Here's how the part is built. I have some questions about the finished solid (model axes, mm). Face numbers are marked on the shaded views. A direction names the side the tool comes from. Coordinates: 2 decimals unless noted, no trailing zeros. Write each loop counter-clockwise with the first axis right and the second up, starting at its lowest first coordinate (ties: lowest second). Pieces come first, ordered by that corner, then holes. Notation, with made-up numbers: (-26, -39) -> (31, -39) arc R18 cw to (31, -15) -> close; hole circle Ø3 at (10, -32.75). An arc over 180 degrees is marked (long way). Put each result on its own line as item: value. Start each with the question number.
Item 1: I need wall thicknesses on line 1 (X direction, y = 17.5, z = 2.5); line 2 (Y direction, x = 0, z = 0.2); line 3 (Y direction, x = 7.5, z = 6.25). Which ranges of each line are inside material? Lowest first, please. Write a range as [from, to].
Item 2: I want a section at A-A, the plane x = 3. List the corners of the cut face in (y, z) for me, then the cut area to 3 significant figures.
Item 3: For pin 1 (11.5 mm diameter, centred on x = 0, y = 17, fed in from +Z); pin 2 (1.3 mm diameter, centred on x = -13, z = 3, fed in from -Y), each with a flat end and sliding along its axis, tell me the tip position at first contact or that it passes through.
Item 4: If we mould it in two halves opening along Y, with no side actions, what happens to the marked faces 3, 4, 5 and 6? For each: released by +Y, released by -Y, zero draft, split by the parting line, or undercut.
Item 5: On a 3-axis mill with a long thin cutter (end or side, diameter ignored), from which of +Z, -Z, +X, -X, +Y, -Y can I reach the whole of each face in a straight line? I mean the marked faces 1 and 2. Say none if no direction works.
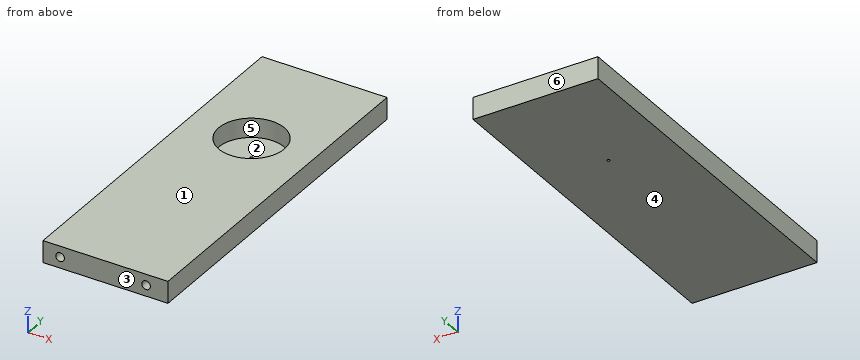
from build123d import *

# Parameters (mm, degrees)
SKETCH1_W                       = 36.27882
SKETCH1_H                       = 102.003225
EXTRUDE1_DEPTH                  = 6.35
SKETCH2_R                       = 9.525
EXTRUDE2_DEPTH                  = 5.588
SKETCH3_R                       = 0.396875
EXTRUDE3_DEPTH                  = 55.419007863
F_3_48_TAPPED_HOLE1_D           = 1.9939
F_3_48_TAPPED_HOLE1_DEPTH       = 9.144
F_3_48_TAPPED_HOLE1_CBORE_D     = 2.5146
F_3_48_TAPPED_HOLE1_CBORE_DEPTH = 7.62
F_3_48_TAPPED_HOLE1_TIP         = 0.599027994


with BuildPart() as part:
    # Sketch1 → Extrude1 (new body)
    with BuildSketch(Plane.XY):
        Rectangle(SKETCH1_W, SKETCH1_H)
    extrude(amount=EXTRUDE1_DEPTH)

    # Sketch2 → Extrude2 (cut)
    with BuildSketch(Plane.XY.offset(6.35)):
        with Locations((0, 17.0005375)):
            Circle(SKETCH2_R)
    extrude(amount=-EXTRUDE2_DEPTH, mode=Mode.SUBTRACT)

    # Sketch3 → Extrude3 (cut, through all)
    with BuildSketch(Plane.XY.offset(0.762)):
        with Locations((0, 17.0005375)):
            Circle(SKETCH3_R)
    extrude(amount=-EXTRUDE3_DEPTH, mode=Mode.SUBTRACT)

    # #3-48 Tapped Hole1
    with Locations(Plane(origin=(-14.071004552, -51.0016125, -59.648711207), x_dir=(0, 0, -1), z_dir=(0, -1, 0))):
        with Locations((-62.823711207, 25.860414552), (-62.823711207, 0.892214552)):
            CounterBoreHole(F_3_48_TAPPED_HOLE1_D / 2, F_3_48_TAPPED_HOLE1_CBORE_D / 2, F_3_48_TAPPED_HOLE1_CBORE_DEPTH, depth=F_3_48_TAPPED_HOLE1_DEPTH)
            with Locations((0, 0, -(F_3_48_TAPPED_HOLE1_DEPTH + F_3_48_TAPPED_HOLE1_TIP / 2))):  # 118° drill point
                Cone(0, F_3_48_TAPPED_HOLE1_D / 2, F_3_48_TAPPED_HOLE1_TIP, mode=Mode.SUBTRACT)


solid = part.part
Calculated:
1. line 1: x = [-18.14, -9.51], [9.51, 18.14]
1. line 2: y = [-51, 16.6], [17.4, 51]
1. line 3: y = [-51, 11.13], [22.87, 51]
2. outline: (-51, 0) -> (51, 0) -> (51, 6.35) -> (26.04, 6.35) -> (26.04, 0.76) -> (7.96, 0.76) -> (7.96, 6.35) -> (-51, 6.35) -> close
2. area: 547 mm2
3. pin 1: stops at z = 0.76
3. pin 2: stops at y = -41.8
4. face 3: released by -Y
4. face 4: zero draft
4. face 5: undercut
4. face 6: released by +Y
5. face 1: +Z, +X, -X, +Y, -Y
5. face 2: +Z
